Check sheet for the modelled part. Datum: model origin and axes. Units: mm. Give positions to 0.01 mm unless a question says otherwise; leave off trailing zeros. Order: outer loops, then holes, each group sorted by start corner. A loop starts at its lowest first (then second) coordinate and runs counter-clockwise, first axis right, second up. Notation, with made-up numbers: (66, 25.25) -> (83, 25.25) arc R21 cw to (83, 35.25) -> close; hole circle Ø6 at (17.25, 69). An arc over 180 degrees is marked (long way). Write each question's results on one line, items separated by ' | '.
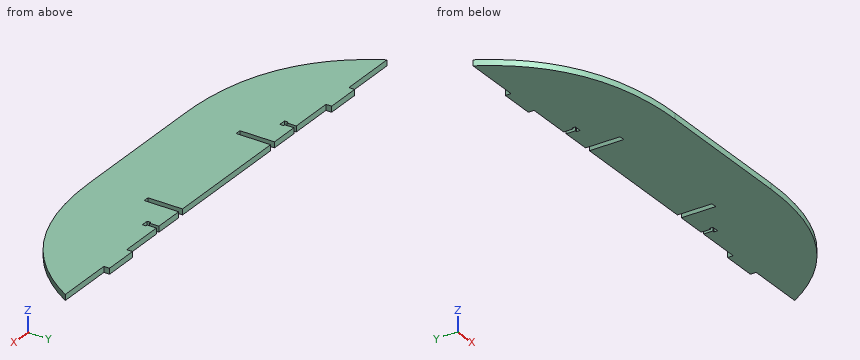
from build123d import *

# Parameters (mm, degrees)
BOSS_EXTRUDE13_DEPTH = 6.35


with BuildPart() as part:
    # Sketch1 → Boss-Extrude13 (new body)
    with BuildSketch(Plane.XY):
        with BuildLine():
            Line((-193.675, 406.4), (-130.538105188, 406.4))
            Line((-130.538105188, 406.4), (-130.538105188, 412.75))
            Line((-130.538105188, 412.75), (-92.438105188, 412.75))
            Line((-92.438105188, 412.75), (-92.438105188, 406.4))
            Line((-92.438105188, 406.4), (-43.316932521, 406.4))
            Line((-43.316932521, 406.4), (-43.316932521, 396.24))
            Line((-43.316932521, 396.24), (-45.221932521, 396.24))
            Line((-45.221932521, 396.24), (-45.221932521, 392.176))
            Line((-45.221932521, 392.176), (-37.347932521, 392.176))
            Line((-37.347932521, 392.176), (-37.347932521, 396.24))
            Line((-37.347932521, 396.24), (-39.252932521, 396.24))
            Line((-39.252932521, 396.24), (-39.252932521, 406.4))
            Line((-39.252932521, 406.4), (-7.076210377, 406.4))
            Line((-7.076210377, 406.4), (-7.076210377, 368.3))
            Line((-7.076210377, 368.3), (-6.35, 368.3))
            Line((-6.35, 368.3), (-0.726210377, 368.3))
            Line((-0.726210377, 368.3), (-0.726210377, 406.4))
            Line((-0.726210377, 406.4), (0, 406.4))
            Line((0, 406.4), (145.323789623, 406.4))
            Line((145.323789623, 406.4), (145.323789623, 368.3))
            Line((145.323789623, 368.3), (151.673789623, 368.3))
            Line((151.673789623, 368.3), (151.673789623, 406.4))
            Line((151.673789623, 406.4), (152.4, 406.4))
            Line((152.4, 406.4), (184.576722144, 406.4))
            Line((184.576722144, 406.4), (184.576722144, 396.24))
            Line((184.576722144, 396.24), (182.671722144, 396.24))
            Line((182.671722144, 396.24), (182.671722144, 392.176))
            Line((182.671722144, 392.176), (190.545722144, 392.176))
            Line((190.545722144, 392.176), (190.545722144, 396.24))
            Line((190.545722144, 396.24), (188.640722144, 396.24))
            Line((188.640722144, 396.24), (188.640722144, 406.4))
            Line((188.640722144, 406.4), (237.761894812, 406.4))
            Line((237.761894812, 406.4), (237.761894812, 412.75))
            Line((237.761894812, 412.75), (275.861894812, 412.75))
            Line((275.861894812, 412.75), (275.861894812, 406.4))
            Line((275.861894812, 406.4), (339.75144841, 406.4))
            add(Edge.make_bspline(
                [(152.4, 307.792730185), (282.8477338, 308.473912291), (339.75144841, 406.4)],
                knots=[0, 0, 0, 1, 1, 1], degree=2))
            Line((152.4, 307.792730185), (-6.35, 307.792730185))
            add(Edge.make_bspline(
                [(-193.675, 406.4), (-138.010339731, 307.440275388), (-6.35, 307.792730185)],
                knots=[0, 0, 0, 1, 1, 1], degree=2))
        make_face()
    extrude(amount=BOSS_EXTRUDE13_DEPTH)


solid = part.part
1. Section check B-B on y = 374.5. Give the number of separate pieces and of enclosed holes in the cut face, then the cut area to 3 significant figures.
Verdict:
separate pieces: 3 | enclosed holes: 0 | area: 3,020 mm^2
2. Material ranges on probe 1 along X at (y, z) = (387.5, 6); probe 2 along X at (y, z) = (401, 2.25); probe 3 along X at (y, z) = (370, 1.25), recorded low to high. Write a range as from..to.
Verdict:
probe 1: x = -181.71..-7.08, -0.73..145.32, 151.67..327.43 | probe 2: x = -190.54..-43.32, -39.25..-7.08, -0.73..145.32, 151.67..184.58, 188.64..336.51 | probe 3: x = -167.66..-7.08, -0.73..145.32, 151.67..313.02
3. Gauge pin test, flat ends, axial feed: pin 1 Ø3 at (y, z) = (388.5, 3.5) entering from -X; pin 2 Ø1 at (y, z) = (336.5, 2) entering from -X; pin 3 Ø1.9 at (y, z) = (409, 4.5) entering from +X. Record the tip position at first contact, or that the pin passes through.
Verdict:
pin 1: stops at x = -183.46 | pin 2: stops at x = -127.44 | pin 3: stops at x = 275.86
4. Section check A-A on x = 82.5. Record the cut outline in (y, z), then the cut area to 3 significant figures.
Verdict:
outline: (307.79, 0) -> (406.4, 0) -> (406.4, 6.35) -> (307.79, 6.35) -> close | area: 626 mm^2
